Verification items for the finished model (mm, model axes). Round coordinates to 2 decimals unless told otherwise and drop trailing zeros. Order: outer loops, then holes, each group sorted by start corner. A loop starts at its lowest first (then second) coordinate and runs counter-clockwise, first axis right, second up. Notation, with made-up numbers: (41.25, 20.5) -> (52.25, 20.5) arc R16 ccw to (52.25, 25.5) -> close; hole circle Ø1 at (57.25, 56). An arc over 180 degrees is marked (long way). Return JSON: item names as keys, results as strings. Group by question number.
1) Section check A-A on y = 135. Enter the section's corners in (x, z).
2) Section check B-B on x = 4.25. Enter the section's corners in (y, z).
3) Draft check along X on faces 1 (the flat face through (-11.75, 74, 0)), 2 (the flat face through (0, 150, 0)), 3 (the cylindrical face through (6.669, 18.794, 0.07)). Enter one of: pulls with the +X half, pulls with the -X half, needs draft (parallel to the pull), parting line crosses it, or undercut.
4) Scan lines: L1, parallel to Y at x = 4.25, z = 2.75; L2, parallel to Y at x = 3, z = 3; L3, parallel to X at y = 131, z = 1.5. Record each from-to range of solid material in increasing order.
5) Section check C-C on z = 1.75. Enter the section's corners in (x, y).
```python
from build123d import *

# Parameters (mm, degrees)
BOSS_EXTRUDE1_DEPTH  = 150
M8_CLEARANCE_HOLE1_D = 9


with BuildPart() as part:
    # Sketch1 → Boss-Extrude1 (new body)
    with BuildSketch(Plane(origin=(0, 0, 0), x_dir=(1, 0, 0), z_dir=(0, 1, 0))):
        with BuildLine():
            Line((-10.75, -5), (11.75, -5))
            Line((11.75, -5), (11.75, 4))
            ThreePointArc((11.75, 4), (11.457106781, 4.707106781), (10.75, 5))
            Line((10.75, 5), (-10.75, 5))
            ThreePointArc((-10.75, 5), (-11.457106781, 4.707106781), (-11.75, 4))
            Line((-11.75, 4), (-11.75, -4))
            ThreePointArc((-11.75, -4), (-11.457106781, -4.707106781), (-10.75, -5))
        make_face()
    extrude(amount=BOSS_EXTRUDE1_DEPTH)

    # M8 Clearance Hole1 (through all)
    with Locations(Plane(origin=(0, 0, -5), x_dir=(-1, 0, 0), z_dir=(0, 0, -1))):
        with Locations((-4.25, 135), (-4.25, 15)):
            Hole(M8_CLEARANCE_HOLE1_D / 2)


solid = part.part
```
Check result:
{
 "1": {"outline": "(-11.75, -4) arc R1 ccw to (-10.75, -5) -> (-0.25, -5) -> (-0.25, 5) -> (-10.75, 5) arc R1 ccw to (-11.75, 4) -> close; (8.75, -5) -> (10.75, -5) arc R1 ccw to (11.75, -4) -> (11.75, 5) -> (8.75, 5) -> close"},
 "2": {"outline": "(0, -5) -> (10.5, -5) -> (10.5, 5) -> (0, 5) -> close; (19.5, -5) -> (130.5, -5) -> (130.5, 5) -> (19.5, 5) -> close; (139.5, -5) -> (150, -5) -> (150, 5) -> (139.5, 5) -> close"},
 "3": {"face 1": "pulls with the -X half", "face 2": "needs draft", "face 3": "undercut"},
 "4": {"L1": "0 to 10.5, 19.5 to 130.5, 139.5 to 150", "L2": "0 to 10.68, 19.32 to 130.68, 139.32 to 150", "L3": "-11.75 to 2.19, 6.31 to 11.75"},
 "5": {"outline": "(-11.75, 0) -> (11.75, 0) -> (11.75, 150) -> (-11.75, 150) -> close; hole circle Ø9 at (4.25, 15); hole circle Ø9 at (4.25, 135)"}
}
